Input: part model. Units: mm. Frame: model coordinates. Face numbers are marked on the shaded views. Coordinates: 2 decimals unless noted, no trailing zeros. Loops run counter-clockwise (first coordinate to the right, second up) from the corner with the lowest first, then second, coordinate; pieces in that order, holes last. Notation, with made-up numbers: (-22, -16) - (19, -16) arc R13 cw to (19, -8) - close; hole circle Ø4 at (10.25, 57.5). An arc over 180 degrees is marked (long way). Write item = value, one per line. Start each with the question number.
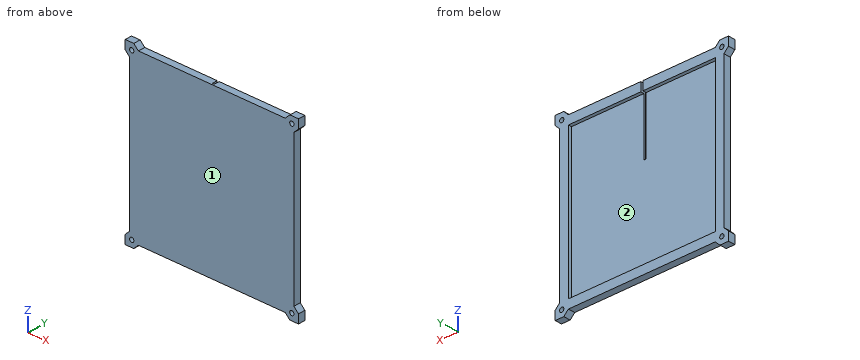
from build123d import *

# Parameters (mm, degrees)
SKETCH1_W            = 380
SKETCH1_H            = 380
BOSS_EXTRUDE1_DEPTH  = 8
SKETCH2_W            = 380
SKETCH2_H            = 380
SKETCH2_W_2          = 340
SKETCH2_H_2          = 340
BOSS_EXTRUDE2_DEPTH  = 8
BOSS_EXTRUDE3_DEPTH  = 16
MIRROR2_COPY_1_DEPTH = 16
SKETCH6_R            = 5
CUT_EXTRUDE1_DEPTH   = 16
SKETCH8_W            = 4.5
SKETCH8_H            = 30
CUT_EXTRUDE2_DEPTH   = 150


with BuildPart() as part:
    # Sketch1 → Boss-Extrude1 (new body)
    with BuildSketch(Plane(origin=(0, 0, 0), x_dir=(1, 0, 0), z_dir=(0, 1, 0))):
        Rectangle(SKETCH1_W, SKETCH1_H)
    extrude(amount=BOSS_EXTRUDE1_DEPTH)

    # Sketch2 → Boss-Extrude2 (add)
    with BuildSketch(Plane(origin=(0, 8, 0), x_dir=(1, 0, 0), z_dir=(0, 1, 0))):
        Rectangle(SKETCH2_W, SKETCH2_H)
        Rectangle(SKETCH2_W_2, SKETCH2_H_2, mode=Mode.SUBTRACT)
    extrude(amount=BOSS_EXTRUDE2_DEPTH)

    # Sketch3 → Boss-Extrude3 (add)
    with BuildSketch(Plane(origin=(0, 16, 0), x_dir=(1, 0, 0), z_dir=(0, 1, 0))):
        Polygon((-200.606601718, 180.606601718), (-190, 170), (-190, 190), (-170, 190), (-180.606601718, 200.606601718), (-200.606601718, 200.606601718), align=None)
    boss_extrude3 = extrude(amount=-BOSS_EXTRUDE3_DEPTH)

    # Mirror1: Boss-Extrude3 across plane
    add(boss_extrude3.mirror(Plane(origin=(0, 0, 0), x_dir=(0, 0, 1), z_dir=(1, 0, 0))))

    # Mirror2: Boss-Extrude3 across plane
    add(boss_extrude3.mirror(Plane.XY))

    # Mirror2 copy 1 sketch → Mirror2 copy 1 (add)
    with BuildSketch(Plane(origin=(0, 16, 0), x_dir=(-1, 0, 0), z_dir=(0, 1, 0))):
        Polygon((-200.606601718, 180.606601718), (-190, 170), (-190, 190), (-170, 190), (-180.606601718, 200.606601718), (-200.606601718, 200.606601718), align=None)
    extrude(amount=-MIRROR2_COPY_1_DEPTH)

    # Sketch6 → Cut-Extrude1 (cut)
    with BuildSketch(Plane(origin=(0, 16, 0), x_dir=(1, 0, 0), z_dir=(0, 1, 0))):
        with Locations(Location((-185.303300859, 185.303300859, 0), (0, 0, 270))):
            Circle(SKETCH6_R)
        with Locations(Location((185.303300859, 185.303300859, 0), (0, 0, 90))):
            Circle(SKETCH6_R)
        with Locations(Location((185.303300859, -185.303300859, 0), (0, 0, 270))):
            Circle(SKETCH6_R)
        with Locations(Location((-185.303300859, -185.303300859, 0), (0, 0, 90))):
            Circle(SKETCH6_R)
    extrude(amount=-CUT_EXTRUDE1_DEPTH, mode=Mode.SUBTRACT)

    # Sketch8 → Cut-Extrude2 (cut)
    with BuildSketch(Plane.XY.offset(190)):
        with Locations((0, 18.75)):
            Rectangle(SKETCH8_W, SKETCH8_H)
    extrude(amount=-CUT_EXTRUDE2_DEPTH, mode=Mode.SUBTRACT)


solid = part.part
Item 1: Pull-direction query (X, two-part tool) for the marked faces 1 and 2; classes: pulls with the +X half, pulls with the -X half, needs draft (parallel to the pull), parting line crosses it, or undercut.
Item 2: Cut plane B-B on y = 12. State how many separate pieces and enclosed holes the cut face has, plus the area to 3 significant figures.
Item 3: Ray query, line 1 (Z direction, x = -52, y = 15); line 2 (X direction, y = 6, z = 137.5). Return the intervals inside material, ascending.
Item 4: Cut plane A-A on z = 50. Return loops of the section in (x, y).
Item 5: Pin query (flat end, axial travel): pin 1 (8 mm diameter, centred on y = 5, z = 75.5, fed in from -X); pin 2 (2.5 mm diameter, centred on y = 11, z = -17, fed in from +X); pin 3 (2.5 mm diameter, centred on x = -61.5, y = 11.5, fed in from +Z); pin 4 (2 mm diameter, centred on x = 68, z = -146, fed in from -Y). Return the tip coordinate at first contact, or that it passes through.
Item 6: Cut plane C-C on x = -90. Return loops of the section in (y, z), plus the area to 3 significant figures.
Recorded:
q1.face_1 = needs draft
q1.face_2 = undercut
q2.separate_pieces = 1
q2.enclosed_holes = 4
q2.area = 30,100 mm²
q3.line_1 = -190 to -170, 170 to 190
q3.line_2 = -190 to -2.25, 2.25 to 190
q4.outline = (-190, 0) - (190, 0) - (190, 16) - (170, 16) - (170, 8) - (2.25, 8) - (2.25, 3.75) - (-2.25, 3.75) - (-2.25, 8) - (-170, 8) - (-170, 16) - (-190, 16) - close
q5.pin_1 = -190
q5.pin_2 = 190
q5.pin_3 = 190
q5.pin_4 = 0
q6.outline = (0, -190) - (16, -190) - (16, -170) - (8, -170) - (8, 170) - (16, 170) - (16, 190) - (0, 190) - close
q6.area = 3,360 mm²
